Autodesk Inventor part; units mm, degrees
ref_plane "YZ Plane" through (0, 0, 0) normal (1, 0, 0) x (0, 1, 0)
ref_plane "XZ Plane" through (0, 0, 0) normal (0, 1, 0) x (-1, 0, 0)
ref_plane "XY Plane" through (0, 0, 0) normal (0, 0, 1) x (1, 0, 0)
sketch "Sketch1" plane through (0, 0, 0) normal (0, 0, 1) x (1, 0, 0)
  circle A0 centre (0, 0) radius 6.5
  circle A1 centre (0, 0) radius 15
  arc A2 (-18.9737, 9) -> (-20.5122, 4.5) centre (0, 0) ccw
  arc A3 (-14.4222, -9) -> (-16.3936, 4.5) centre (0, 0) ccw
  line L0 (0, 17) -> (-4.5, 17) construction
  line L1 (17, 0) -> (17, -4.5) construction
  line L2 (16.3936, -4.5) -> (14.3091, -4.5)
  line L3 (0, -17) -> (4.5, -17) construction
  line L4 (4.5, -16.3936) -> (4.5, -14.3091)
  line L5 (-17, 0) -> (-17, 4.5) construction
  line L6 (-17, 4.5) -> (-14.3091, 4.5)
  line L7 (0, 0) -> (-100, 0) construction
  arc A4 (-100, 9) -> (-100, -9) centre (-100, 0) ccw
  line L8 (-100, -9) -> (-12, -9)
  line L9 (-100, 9) -> (-18.9737, 9)
  line L10 (-14.4222, 9) -> (-12, 9)
  line L11 (-17, 4.5) -> (-20.5122, 4.5)
  line L12 (-4.5, 16.3936) -> (-4.5, 14.3091)
  line L13 (-4.5, 16.3936) -> (-4.5, 17) construction
  line L14 (17, -4.5) -> (16.3936, -4.5) construction
  line L15 (4.5, -17) -> (4.5, -16.3936) construction
  circle A5 centre (0, 0) radius 21
  line L16 (-4.5, 16.3936) -> (-4.5, 20.5122)
  line L17 (4.5, -16.3936) -> (4.5, -20.5122)
  line L18 (16.3936, -4.5) -> (20.5122, -4.5)
  dimension "d3" = 34
  dimension "d0" = 13
  dimension "d1" = 30
  dimension "d2" = 42
  dimension "d4" = 4.5
  dimension "d5" = 4.5
  dimension "d6" = 4.5
  dimension "d7" = 4.5
  dimension "d8" = 100
  dimension "d9" = 9
extrude "Extrusion1" add sketch "Sketch1" along normal blind 9 contours A1 | A1 L10 A3 L12 | L2 A3 L4 A1 | A1 L6 A3 L10 | A1 L8 A5 L11 L6 | A2 A5 L8 A4 L9
extrude "Extrusion2" add sketch "Sketch1" along normal blind 15.5 and the other way blind 6.5 contours A3 L6 L11 A2 A5 L16 | L18 A5 L17 A3
sketch "Sketch2" plane through (-100, -9, 0) normal (0, -1, 0) x (1, 0, 0)
  line L0 (0, 0) -> (134.8199, 0) construction
  line L1 (100, 0) -> (100, -17.6353) construction
  line L2 (100, 0) -> (104.5, 0) construction
  line L3 (115, 0) -> (95.5, 0) construction
  line L4 (100, 0) -> (100, 4.5) construction
  circle A0 centre (100, 4.5) radius 2
  point P0 (114.3091, 0)
  dimension "d25" = 4.5
  dimension "d26" = 4.5
  dimension "d27" = 4
extrude "Extrusion3" cut sketch "Sketch2" along normal mid plane 89
equation "\"d5\" = d4"
equation "\"d6\" = d4"
equation "\"d7\" = d4"
properties part number "Handle" material "Steel, Mild"
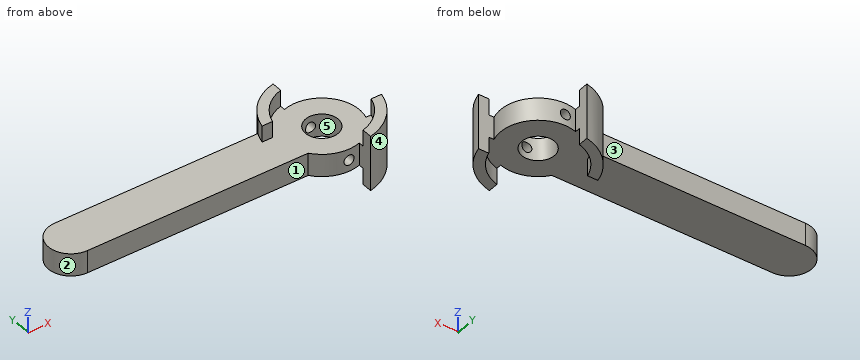
Geometry: final body of the model. Coordinates: model frame, mm. Face numbers are marked on the shaded views. A direction names the side the tool comes from. Round coordinates to 2 decimals unless told otherwise and drop trailing zeros. Write each loop counter-clockwise with the first axis right and the second up, starting at its lowest first coordinate (ties: lowest second). Pieces come first, ordered by that corner, then holes. Notation, with made-up numbers: M 71.25,-25 L 97.25,-25 A24 cw 97.25,0 Z; hole C 54.5,80 d11. An arc over 180 degrees is marked long. Answer in a Markdown table with one row per item. Add a question column.
(1) Draft query along Y for the marked faces 3, 4 and 5. Return one class per face: pulls with the +Y half, pulls with the -Y half, needs draft (parallel to the pull), parting line crosses it, or undercut.
(2) Contact query for flat-ended pins moving along their axis: pin 1 (5 mm diameter, centred on x = 0, z = 4.5, fed in from +Y); pin 2 (3 mm diameter, centred on x = -9, y = 2, fed in from +Z); pin 3 (4 mm diameter, centred on y = 4, z = 1.5, fed in from +X). Output: stop coordinate, or through.
(3) Cut plane B-B, the plane x = 0. Return the cut outline in (y, z), then the cut area to 3 significant figures.
(4) Cut plane C-C, the plane z = 13. Return the cut outline in (x, y).
(5) Reachability of the marked faces 1 and 2 from +Z, -Z, +X, -X, +Y, -Y: full face, straight path, thin tool, end or side. Return the list, or none.
(6) Cut plane D-D, the plane y = -13. Return the cut outline in (x, z).
(7) Cut plane A-A, the plane y = 0. Return the cut outline in (x, z), then the cut area to 3 significant figures.
(8) Ray query, L1, parallel to Z at x = 0, y = -10; L2, parallel to X at y = -11.5, z = 3; L3, parallel to Z at x = -74.5, y = 4. Return the intervals inside material, ascending.
Established:
| question | item | result |
|---|---|---|
| 1 | face 3 | pulls with the +Y half |
| 1 | face 4 | pulls with the -Y half |
| 1 | face 5 | undercut |
| 2 | pin 1 | y = 15 |
| 2 | pin 2 | z = 9 |
| 2 | pin 3 | x = 14.87 |
| 3 | outline | M -15,0 L -6.5,0 L -6.5,2.5 L -15,2.5 Z; M -15,6.5 L -6.5,6.5 L -6.5,9 L -15,9 Z; M 6.5,0 L 15,0 L 15,2.5 L 6.5,2.5 Z; M 6.5,6.5 L 15,6.5 L 15,9 L 6.5,9 Z |
| 3 | area | 85.0 mm² |
| 4 | outline | M -20.51,4.5 L -16.39,4.5 A17 cw -4.5,16.39 L -4.5,20.51 A21 ccw -18.97,9 A21 ccw Z; M 4.5,-20.51 A21 ccw 20.51,-4.5 L 16.39,-4.5 A17 cw 4.5,-16.39 Z |
| 5 | face 1 | +Z, -Z, -X, -Y |
| 5 | face 2 | +Z, -Z, -X |
| 6 | outline | M -7.48,0 L 10.95,0 L 10.95,-6.5 L 16.49,-6.5 L 16.49,15.5 L 10.95,15.5 L 10.95,9 L -7.48,9 Z; hole C 0,4.5 d4 |
| 7 | outline | M -109,0 L -6.5,0 L -6.5,9 L -109,9 Z; M 6.5,0 L 15,0 L 15,9 L 6.5,9 Z |
| 7 | area | 999 mm² |
| 8 | L1 | 0 to 2.5, 6.5 to 9 |
| 8 | L2 | -9.63 to -1.32, 1.32 to 17.57 |
| 8 | L3 | 0 to 9 |
